```python
from build123d import *

# Parameters (mm, degrees)
BOSS_EXTRUDE1_DEPTH = 95.25
LPATTERN1_COUNT     = 2
LPATTERN1_PITCH     = 171.45
LPATTERN2_COUNT     = 2
LPATTERN2_PITCH     = 103.378


with BuildPart() as part:
    # Sketch1 → Boss-Extrude1 (new, symmetric)
    with BuildSketch(Plane.XY):
        Polygon((41.91, 6.731), (48.514, 6.731), (48.514, 50.419), (50.038, 50.419), (50.038, 6.731), (56.388, 6.731), (56.388, 50.419), (57.15, 50.419), (57.15, 6.731), (57.15, -6.731), (-57.15, -6.731), (-57.15, 6.731), (-57.15, 50.419), (-55.626, 50.419), (-55.626, 6.731), (-49.022, 6.731), (-49.022, 50.419), (-47.498, 50.419), (-47.498, 6.731), (-40.894, 6.731), (-40.894, 50.419), (-39.37, 50.419), (-39.37, 6.731), (-32.766, 6.731), (-32.766, 50.419), (-31.242, 50.419), (-31.242, 6.731), (-24.638, 6.731), (-24.638, 50.419), (-23.114, 50.419), (-23.114, 6.731), (-16.51, 6.731), (-16.51, 50.419), (-14.986, 50.419), (-14.986, 6.731), (-8.382, 6.731), (-8.382, 50.419), (-6.858, 50.419), (-6.858, 6.731), (-0.254, 6.731), (-0.254, 50.419), (1.27, 50.419), (1.27, 6.731), (7.874, 6.731), (7.874, 50.419), (9.398, 50.419), (9.398, 6.731), (16.002, 6.731), (16.002, 50.419), (17.526, 50.419), (17.526, 6.731), (24.13, 6.731), (24.13, 50.419), (25.654, 50.419), (25.654, 6.731), (32.258, 6.731), (32.258, 50.419), (33.782, 50.419), (33.782, 6.731), (40.386, 6.731), (40.386, 50.419), (41.91, 50.419), align=None)
    extrude(amount=BOSS_EXTRUDE1_DEPTH, both=True)

    # Sketch3 → #8-32 Tapped Hole1 (revolve, cut)
    with BuildSketch(Plane(origin=(47.625, -6.731, 85.725), x_dir=(0, 0, -1), z_dir=(1, 0, 0))):
        Polygon((0, 0), (0, 12.975806461), (1.7272, 11.938), (1.7272, 0), align=None)
    f_8_32_tapped_hole1 = revolve(axis=Axis((47.625, -13.081, 85.725), (0, 1, 0)), mode=Mode.SUBTRACT)

    # Sketch5 → #4-40 Tapped Hole1 (revolve, cut)
    with BuildSketch(Plane(origin=(38.989, -6.731, 25.908), x_dir=(0, 0, -1), z_dir=(1, 0, 0))):
        Polygon((0, 0), (0, 11.855152758), (1.1303, 11.176), (1.1303, 0), align=None)
    f_4_40_tapped_hole1 = revolve(axis=Axis((38.989, -13.081, 25.908), (0, 1, 0)), mode=Mode.SUBTRACT)

    # LPattern1: #8-32 Tapped Hole1 ×2
    with Locations(*[(0, 0, -i * LPATTERN1_PITCH) for i in range(1, LPATTERN1_COUNT)]):
        add(f_8_32_tapped_hole1, mode=Mode.SUBTRACT)

    # LPattern2: #4-40 Tapped Hole1 ×2
    with Locations(*[(0, 0, -i * LPATTERN2_PITCH) for i in range(1, LPATTERN2_COUNT)]):
        add(f_4_40_tapped_hole1, mode=Mode.SUBTRACT)

    # Mirror1: #8-32 Tapped Hole1, #4-40 Tapped Hole1 across plane
    add(f_8_32_tapped_hole1.mirror(Plane(origin=(0, 0, 0), x_dir=(0, 0, 1), z_dir=(1, 0, 0))), mode=Mode.SUBTRACT)
    add(f_4_40_tapped_hole1.mirror(Plane(origin=(0, 0, 0), x_dir=(0, 0, 1), z_dir=(1, 0, 0))), mode=Mode.SUBTRACT)

    # Mirror1 copy 1 sketch → Mirror1 copy 1 (revolve, cut)
    with BuildSketch(Plane(origin=(-47.625, -6.731, -85.725), x_dir=(0, 0, -1), z_dir=(-1, 0, 0))):
        Polygon((0, 0), (0, -12.975806461), (1.7272, -11.938), (1.7272, 0), align=None)
    revolve(axis=Axis((-47.625, -13.081, -85.725), (0, -1, 0)), mode=Mode.SUBTRACT)

    # Mirror1 copy 2 sketch → Mirror1 copy 2 (revolve, cut)
    with BuildSketch(Plane(origin=(-38.989, -6.731, -77.47), x_dir=(0, 0, -1), z_dir=(-1, 0, 0))):
        Polygon((0, 0), (0, -11.855152758), (1.1303, -11.176), (1.1303, 0), align=None)
    revolve(axis=Axis((-38.989, -13.081, -77.47), (0, -1, 0)), mode=Mode.SUBTRACT)


solid = part.part
```
Read the model definition and answer for the solid it produces. Units are mm, in the model's axes. A direction names the side the tool comes from. Round coordinates to 2 decimals unless told otherwise and drop trailing zeros. Answer in a Markdown table with one row per item. Add a question column.
1) Find section A-A, the plane y = 42. State how many separate pieces and enclosed holes the cut face has, and give its area (3 significant figures).
2) Determine the mould class of faces 3 (the face through (57.15, 21, 1)), 4 (the face through (1, 10, 95.25)), 5 (the face through (32.258, 28, 1)) for opening direction X: pulls with the +X half, pulls with the -X half, needs draft (parallel to the pull), parting line crosses it, or undercut.
3) Which of the six approach directions +Z, -Z, +X, -X, +Y, -Y give full straight-line access (tool end or side, diameter ignored) to faces 1 (the face through (47.535, 6.065, 85.439)), 2 (the face through (25.654, 29, 1))?
4) Consider line 1 (Z direction, x = 48, y = 5); line 2 (X direction, y = 0.5, z = -77.47); line 3 (X direction, y = -3.5, z = 25). Determine where each line is inside the solid, lowest interval first.
5) Given P1, Ø5.5, axis at x = -53, z = -29.5, coming from the +Y side; P2, Ø1.9, axis at x = 53, z = 19.5, coming from the +Y side, each flat-ended and moving along its own axis, determine where each tip first touches the part or whether it passes through.
Findings below:
| question | item | result |
|---|---|---|
| 1 | separate pieces | 15 |
| 1 | enclosed holes | 0 |
| 1 | area | 4,210 mm² |
| 2 | face 3 | pulls with the +X half |
| 2 | face 4 | needs draft |
| 2 | face 5 | undercut |
| 3 | face 1 | -Y |
| 3 | face 2 | +Z, -Z, +Y |
| 4 | line 1 | -95.25 to -87.41, -84.04 to 84.04, 87.41 to 95.25 |
| 4 | line 2 | -57.15 to -40.12, -37.86 to 37.86, 40.12 to 57.15 |
| 4 | line 3 | -57.15 to -39.66, -38.32 to 38.32, 39.66 to 57.15 |
| 5 | P1 | y = 50.42 |
| 5 | P2 | y = 6.73 |
